Verification items for this drawing (mm, ordinates from the low corner). A direction names the side the tool comes from. Round coordinates to 2 decimals unless told otherwise and drop trailing zeros. Order: outer loops, then holes, each group sorted by start corner. A loop starts at its lowest first (then second) coordinate and runs counter-clockwise, first axis right, second up. Notation, with made-up numbers: (-9, -18) -> (10, -18) arc R16 cw to (10, -12) -> close; hole circle Ø5 at (-13, 31). An arc over 180 degrees is marked (long way). Use a Markdown table: item, result. Add a question column.
Item 1: Sectioned sample at D-D, the plane x = 24. Record the cut outline in (y, z).
Item 2: Gauge pin test, flat end, axial feed: pin 1 Ø3 at (x, y) = (28, 7) entering from +Z. Record the tip position at first contact, or that the pin passes through.
Item 3: Set-up check for the marked faces 1 and 2: record each of +Z, -Z, +X, -X, +Y, -Y from which the full face is reachable in a straight line by a thin tool's end or side.
Item 4: Sectioned sample at C-C, the plane y = 13.5. Record the cut outline in (x, z), and give its area (3 significant figures).
Item 5: Sectioned sample at A-A, the plane y = 37. Record the cut outline in (x, z), and give its area (3 significant figures).
Item 6: Sectioned sample at B-B, the plane x = 52.5. Record the cut outline in (y, z), and give its area (3 significant figures).
Item 7: Material ranges on probe 1 along Z at (x, y) = (57, 6.5), recorded low to high. Write a range as [from, to].
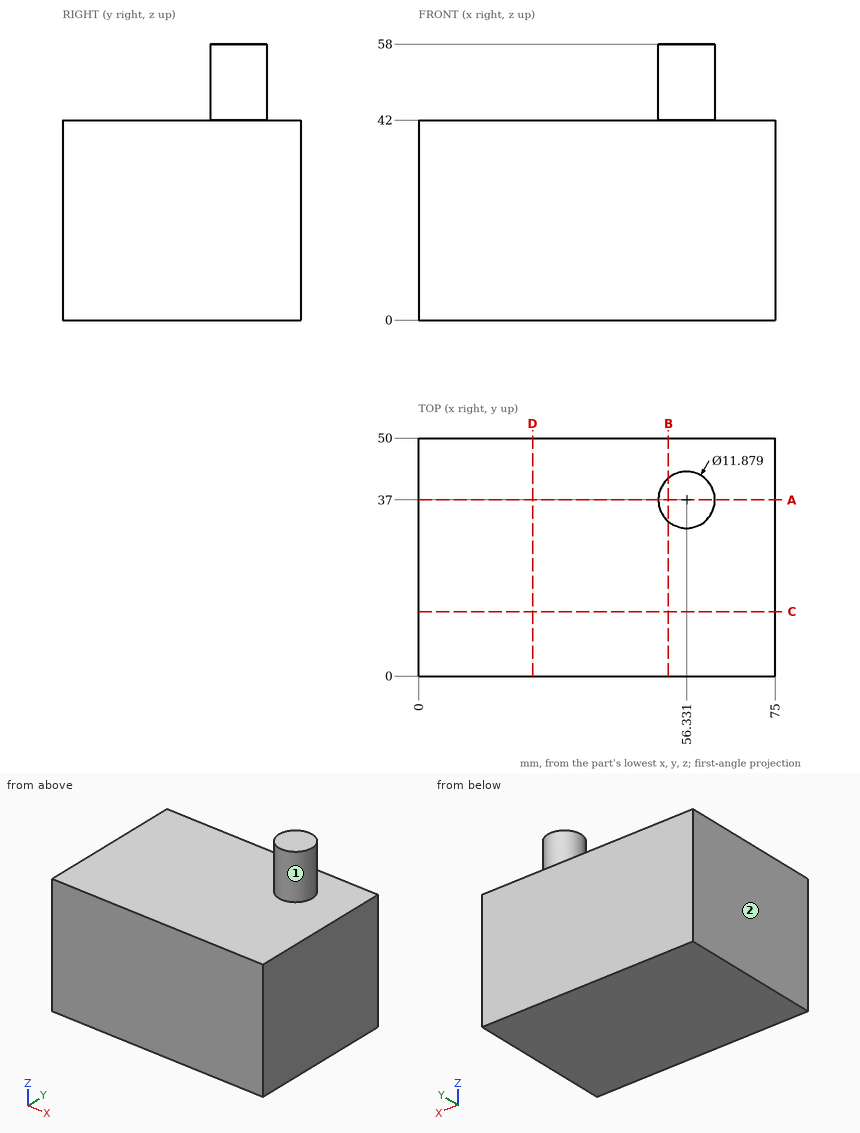
Found:
| question | item | result |
|---|---|---|
| 1 | outline | (0, 0) -> (50, 0) -> (50, 42) -> (0, 42) -> close |
| 2 | pin 1 | stops at z = 42 |
| 3 | face 1 | +Z |
| 3 | face 2 | +Z, -Z, -X, +Y, -Y |
| 4 | outline | (0, 0) -> (75, 0) -> (75, 42) -> (0, 42) -> close |
| 4 | area | 3,150 mm2 |
| 5 | outline | (0, 0) -> (75, 0) -> (75, 42) -> (62.27, 42) -> (62.27, 58) -> (50.39, 58) -> (50.39, 42) -> (0, 42) -> close |
| 5 | area | 3,340 mm2 |
| 6 | outline | (0, 0) -> (50, 0) -> (50, 42) -> (41.54, 42) -> (41.54, 58) -> (32.46, 58) -> (32.46, 42) -> (0, 42) -> close |
| 6 | area | 2,250 mm2 |
| 7 | probe 1 | z = [0, 42] |
